Build history of the part. All positions in model axes, mm. A direction names the side the tool comes from. Round coordinates to 2 decimals unless told otherwise and drop trailing zeros. Loops run counter-clockwise (first coordinate to the right, second up) from the corner with the lowest first, then second, coordinate; pieces in that order, holes last. Notation, with made-up numbers: (-3.75, -27) - (49.25, -27) arc R18 cw to (49.25, -23) - close; hole circle Ø6 at (-29, 25.5). An arc over 180 degrees is marked (long way). Use a Markdown table: item, result.
from build123d import *

# Parameters (mm, degrees)
PAD_DEPTH    = 19
FILLET_R     = 5
FILLET001_R  = 1
SKETCH001_R  = 2
POCKET_DEPTH = 127.001


with BuildPart() as part:
    # Sketch → Pad (new body)
    with BuildSketch(Plane.XY):
        Polygon((-104.21047, 0), (-99.21047, 0), (-99.21047, 52), (17.78953, 52), (17.78953, 0), (22.78953, 0), (22.78953, 60), (-104.21047, 60), align=None)
    extrude(amount=PAD_DEPTH)

    # Fillet
    fillet_edges = [part.edges().sort_by_distance(p)[0] for p in [
        (-101.71047, 0, 0),
        (20.28953, 0, 0),
    ]]
    fillet(fillet_edges, radius=FILLET_R)

    # Fillet001
    fillet001_edges = [part.edges().sort_by_distance(p)[0] for p in [
        (-40.71047, 52, 0),
        (17.78953, 28.5, 0),
        (-99.21047, 28.5, 0),
        (-99.21047, 26, 19),
        (-40.71047, 52, 19),
        (-104.21047, 32.5, 0),
        (-40.71047, 60, 0),
        (22.78953, 32.5, 0),
        (22.78953, 1.464466, 1.464466),
        (17.78953, 1.464466, 1.464466),
        (22.78953, 30, 19),
        (22.78953, 60, 9.5),
        (-40.71047, 60, 19),
        (-104.21047, 60, 9.5),
        (17.78953, 26, 19),
        (20.28953, 0, 19),
        (-101.71047, 0, 19),
        (-104.21047, 0, 12),
        (-99.21047, 0, 12),
        (-104.21047, 30, 19),
        (22.78953, 0, 12),
        (17.78953, 0, 12),
        (-104.21047, 1.464466, 1.464466),
        (-99.21047, 1.464466, 1.464466),
    ]]
    fillet(fillet001_edges, radius=FILLET001_R)

    # Sketch001 → Pocket (cut, through all)
    with BuildSketch(Plane.YZ.offset(22.78953)):
        with Locations((9.5, 9.5)):
            Circle(SKETCH001_R)
    extrude(amount=-POCKET_DEPTH, mode=Mode.SUBTRACT)


solid = part.part
Q1. Which spindle directions (+Z, -Z, +X, -X, +Y, -Y) get a long thin tool onto all of the face, cutting with end or side? Do faces 5 (the face through (-41, 54, 0)), 6 (the face through (-99.21, 26, 9)). Say none if no direction does.
Results found:
| item | result |
|---|---|
| face 5 | -Z, +X, -X, +Y, -Y |
| face 6 | +Z, -Z, -Y |
Q2. Cut at A-A, the plane y = 9.5. List the corners of the cut face in (x, z), plus the area to 3 significant figures.
Results found:
| item | result |
|---|---|
| outline | (-104.21, 1) arc R1 ccw to (-103.21, 0) - (-100.21, 0) arc R1 ccw to (-99.21, 1) - (-99.21, 7.5) - (-104.21, 7.5) - close; (-104.21, 11.5) - (-99.21, 11.5) - (-99.21, 18) arc R1 ccw to (-100.21, 19) - (-103.21, 19) arc R1 ccw to (-104.21, 18) - close; (17.79, 1) arc R1 ccw to (18.79, 0) - (21.79, 0) arc R1 ccw to (22.79, 1) - (22.79, 7.5) - (17.79, 7.5) - close; (17.79, 11.5) - (22.79, 11.5) - (22.79, 18) arc R1 ccw to (21.79, 19) - (18.79, 19) arc R1 ccw to (17.79, 18) - close |
| area | 148 mm2 |
Q3. Pull direction Z, two halves, no side cores. Call faces 1 (the face through (-101.675, 9.24, 11.483)), 2 (the face through (20.325, 9.24, 11.483)), 3 (the face through (-41, 54, 19)), 4 (the face through (17.79, 27, 9)): pulls with the +Z half, pulls with the -Z half, needs draft (parallel to the pull), parting line crosses it, or undercut.
Results found:
| item | result |
|---|---|
| face 1 | undercut |
| face 2 | undercut |
| face 3 | pulls with the +Z half |
| face 4 | needs draft |
Q4. Cut at C-C, the plane y = 44.5. List the corners of the cut face in (x, z).
Results found:
| item | result |
|---|---|
| outline | (-104.21, 1) arc R1 ccw to (-103.21, 0) - (-100.21, 0) arc R1 ccw to (-99.21, 1) - (-99.21, 18) arc R1 ccw to (-100.21, 19) - (-103.21, 19) arc R1 ccw to (-104.21, 18) - close; (17.79, 1) arc R1 ccw to (18.79, 0) - (21.79, 0) arc R1 ccw to (22.79, 1) - (22.79, 18) arc R1 ccw to (21.79, 19) - (18.79, 19) arc R1 ccw to (17.79, 18) - close |
Q5. Cut at B-B, the plane z = 9.5. List the corners of the cut face in (x, y).
Results found:
| item | result |
|---|---|
| outline | (-104.21, 1) arc R1 ccw to (-103.21, 0) - (-100.21, 0) arc R1 ccw to (-99.21, 1) - (-99.21, 7.5) - (-104.21, 7.5) - close; (-104.21, 11.5) - (-99.21, 11.5) - (-99.21, 52) - (17.79, 52) - (17.79, 11.5) - (22.79, 11.5) - (22.79, 59) arc R1 ccw to (21.79, 60) - (-103.21, 60) arc R1 ccw to (-104.21, 59) - close; (17.79, 1) arc R1 ccw to (18.79, 0) - (21.79, 0) arc R1 ccw to (22.79, 1) - (22.79, 7.5) - (17.79, 7.5) - close |
Q6. Drop flat-ended pins along their axis: pin 1 (3 mm diameter, centred on x = 7.5, y = 51, fed in from -Z); pin 2 (8.5 mm diameter, centred on x = -13, z = 13, fed in from -Y); pin 3 (3 mm diameter, centred on y = 9.5, z = 9.5, fed in from -X). Give the stop position or say it passes through.
Results found:
| item | result |
|---|---|
| pin 1 | stops at z = 0.13 |
| pin 2 | stops at y = 52 |
| pin 3 | passes through |
Q7. Cut at D-D, the plane x = -35. List the corners of the cut face in (y, z), plus the area to 3 significant figures.
Results found:
| item | result |
|---|---|
| outline | (52, 1) arc R1 ccw to (53, 0) - (59, 0) arc R1 ccw to (60, 1) - (60, 18) arc R1 ccw to (59, 19) - (53, 19) arc R1 ccw to (52, 18) - close |
| area | 151 mm2 |
Q8. Probe line 1 (X direction, y = 24, z = 4.25); line 2 (Y direction, x = -90, z = 4); line 3 (Z direction, x = 21, y = 9). List the from-to ranges inside material, lowest first.
Results found:
| item | result |
|---|---|
| line 1 | x = -104.21 to -99.21, 17.79 to 22.79 |
| line 2 | y = 52 to 60 |
| line 3 | z = 0 to 7.56, 11.44 to 19 |
